Build history of the part. All positions in model axes, mm. A direction names the side the tool comes from. Give positions to 0.01 mm unless a question says otherwise; leave off trailing zeros. Order: outer loops, then holes, each group sorted by start corner. A loop starts at its lowest first (then second) coordinate and runs counter-clockwise, first axis right, second up. Notation, with made-up numbers: M 20.25,79 L 53.25,79 A29 cw 53.25,118 Z; hole C 32.25,-6.75 d3. An arc over 180 degrees is marked long. One line per item, written item: value.
from build123d import *

# Parameters (mm, degrees)
F0_R     = 2.5
F1_DEPTH = 2
F2_DEPTH = 25


# Not quite as in the source:
# - a feature names something its author has since deleted; it is built from what else it names


with BuildPart() as f1:
    # F0 (on Top) → F1 (new body)
    with BuildSketch(Plane.XY):
        with BuildLine():
            ThreePointArc((40, 39), (39.2928932188, 39.2928932188), (39, 40))
            Line((39, 40), (20.6155281281, 40))
            ThreePointArc((20.6155281281, 40), (31.8198051534, 31.8198051534), (40, 20.6155281281))
            Line((40, 20.6155281281), (40, 39))
        make_face()
        with BuildLine():
            ThreePointArc((-40, 20.6155281281), (-31.8198051534, 31.8198051534), (-20.6155281281, 40))
            Line((-20.6155281281, 40), (-39, 40))
            ThreePointArc((-39, 40), (-39.2928932188, 39.2928932188), (-40, 39))
            Line((-40, 39), (-40, 20.6155281281))
        make_face()
        with BuildLine():
            ThreePointArc((-20.6155281281, -40), (-31.8198051534, -31.8198051534), (-40, -20.6155281281))
            Line((-40, -20.6155281281), (-40, -39))
            ThreePointArc((-40, -39), (-39.2928932188, -39.2928932188), (-39, -40))
            Line((-39, -40), (-20.6155281281, -40))
        make_face()
        with BuildLine():
            Line((40, -39), (40, -20.6155281281))
            ThreePointArc((40, -20.6155281281), (31.8198051534, -31.8198051534), (20.6155281281, -40))
            Line((20.6155281281, -40), (39, -40))
            ThreePointArc((39, -40), (39.2928932188, -39.2928932188), (40, -39))
        make_face()
        with BuildLine():
            ThreePointArc((40, 20.6155281281), (31.8198051534, 31.8198051534), (20.6155281281, 40))
            ThreePointArc((20.6155281281, 40), (0, 45), (-20.6155281281, 40))
            ThreePointArc((-20.6155281281, 40), (-31.8198051534, 31.8198051534), (-40, 20.6155281281))
            ThreePointArc((-40, 20.6155281281), (-45, 0), (-40, -20.6155281281))
            ThreePointArc((-40, -20.6155281281), (-31.8198051534, -31.8198051534), (-20.6155281281, -40))
            ThreePointArc((-20.6155281281, -40), (0, -45), (20.6155281281, -40))
            ThreePointArc((20.6155281281, -40), (31.8198051534, -31.8198051534), (40, -20.6155281281))
            ThreePointArc((40, -20.6155281281), (43.7321392113, -10.6066017178), (45, 0))
            ThreePointArc((45, 0), (43.7321392113, 10.6066017178), (40, 20.6155281281))
        make_face()
        Circle(F0_R, mode=Mode.SUBTRACT)
        with BuildLine():
            Line((-40, 40), (-39, 40))
            ThreePointArc((-39, 40), (-40.7071067812, 40.7071067812), (-40, 39))
            Line((-40, 39), (-40, 40))
        make_face()
        with BuildLine():
            ThreePointArc((-40, 39), (-39.2928932188, 39.2928932188), (-39, 40))
            Line((-39, 40), (-40, 40))
            Line((-40, 40), (-40, 39))
        make_face()
        with BuildLine():
            Line((40, 40), (39, 40))
            ThreePointArc((39, 40), (39.2928932188, 39.2928932188), (40, 39))
            Line((40, 39), (40, 40))
        make_face()
        with BuildLine():
            ThreePointArc((40, 39), (40.7071067812, 39.2928932188), (41, 40))
            ThreePointArc((41, 40), (40, 41), (39, 40))
            Line((39, 40), (40, 40))
            Line((40, 40), (40, 39))
        make_face()
        with BuildLine():
            ThreePointArc((41, -40), (40.7071067812, -39.2928932188), (40, -39))
            Line((40, -39), (40, -40))
            Line((40, -40), (39, -40))
            ThreePointArc((39, -40), (40, -41), (41, -40))
        make_face()
        with BuildLine():
            Line((40, -40), (40, -39))
            ThreePointArc((40, -39), (39.2928932188, -39.2928932188), (39, -40))
            Line((39, -40), (40, -40))
        make_face()
        with BuildLine():
            Line((-40, -40), (-40, -39))
            ThreePointArc((-40, -39), (-40.7071067812, -40.7071067812), (-39, -40))
            Line((-39, -40), (-40, -40))
        make_face()
        with BuildLine():
            ThreePointArc((-39, -40), (-39.2928932188, -39.2928932188), (-40, -39))
            Line((-40, -39), (-40, -40))
            Line((-40, -40), (-39, -40))
        make_face()
    extrude(amount=F1_DEPTH)

    # F0 (on Top) → F2 (join)
    with BuildSketch(Plane.XY):
        with BuildLine():
            ThreePointArc((40, 20.6155281281), (31.8198051534, 31.8198051534), (20.6155281281, 40))
            ThreePointArc((20.6155281281, 40), (0, 45), (-20.6155281281, 40))
            ThreePointArc((-20.6155281281, 40), (-31.8198051534, 31.8198051534), (-40, 20.6155281281))
            ThreePointArc((-40, 20.6155281281), (-45, 0), (-40, -20.6155281281))
            ThreePointArc((-40, -20.6155281281), (-31.8198051534, -31.8198051534), (-20.6155281281, -40))
            ThreePointArc((-20.6155281281, -40), (0, -45), (20.6155281281, -40))
            ThreePointArc((20.6155281281, -40), (31.8198051534, -31.8198051534), (40, -20.6155281281))
            ThreePointArc((40, -20.6155281281), (43.7321392113, -10.6066017178), (45, 0))
            ThreePointArc((45, 0), (43.7321392113, 10.6066017178), (40, 20.6155281281))
        make_face()
        Circle(F0_R, mode=Mode.SUBTRACT)
    extrude(amount=F2_DEPTH)


solid = f1.part
1) Drill centre lines: probe 1 along Y at (x, z) = (0, 8); probe 2 along Z at (x, y) = (33.5, 38.5); probe 3 along Y at (x, z) = (-1, 8.25). Where is each one in solid material? Low to high. Write a range as from..to.
Check values:
probe 1: -45..-2.5, 2.5..45
probe 2: 0..2
probe 3: -44.99..-2.29, 2.29..44.99
2) Pin check, flat tips, straight feed: pin 1 (2 mm diameter, centred on x = 27, z = 1, fed in from +Y); pin 2 (1.5 mm diameter, centred on x = 11.5, z = 3, fed in from -Y); pin 3 (12 mm diameter, centred on y = 13.5, z = 17, fed in from -X). Stop position of each tip, or through.
Check values:
pin 1: y = 40
pin 2: y = -43.7
pin 3: x = -44.37
3) Tool access for faces 5 (the face through (30, -40, 1)), 6 (the face through (-30, 40, 1)), 7 (the face through (-40, -30, 1)), 8 (the face through (-33, -35, 2)): list every direction of +Z, -Z, +X, -X, +Y, -Y with a clear straight run to the whole face (end or side of a thin tool).
Check values:
face 5: +Z, -Z, -Y
face 6: +Z, -Z, +Y
face 7: +Z, -Z, -X
face 8: +Z, -X, -Y
4) Saw through at A-A, the plane x = 0. Write the cut outline in (y, z).
Check values:
outline: M -45,0 L -2.5,0 L -2.5,25 L -45,25 Z; M 2.5,0 L 45,0 L 45,25 L 2.5,25 Z
5) Mould opens along X. For faces 1 (the face through (30, 40, 1)), 2 (the face through (-40.683, 40.73, 0.986)), 3 (the face through (40, -30, 1)), 4 (the face through (-1, -9, 25)) say: released by +X, released by -X, zero draft, split by the parting line, or undercut.
Check values:
face 1: undercut
face 2: undercut
face 3: released by +X
face 4: zero draft
6) Saw through at D-D, the plane x = -25. Write the cut outline in (y, z).
Check values:
outline: M -40,0 L 40,0 L 40,2 L 37.42,2 L 37.42,25 L -37.42,25 L -37.42,2 L -40,2 Z
7) Saw through at C-C, the plane z = 6.5. Write the cut outline in (x, y).
Check values:
outline: C 0,0 d90; hole C 0,0 d5
